```python
from build123d import *

# Parameters (mm, degrees)
SKETCH1_W           = 67
SKETCH1_H           = 40
BOSS_EXTRUDE1_DEPTH = 2
SKETCH2_W           = 55
SKETCH2_H           = 40
BOSS_EXTRUDE2_DEPTH = 2
SKETCH3_W           = 49
SKETCH3_H           = 38
BOSS_EXTRUDE4_DEPTH = 1
CUT_EXTRUDE1_REACH  = 80.09
SKETCH4_R           = 1.5
CUT_EXTRUDE2_REACH  = 80.09
SKETCH5_R           = 1.5
CUT_EXTRUDE3_REACH  = 80.09
SKETCH6_R           = 1.5
CUT_EXTRUDE4_REACH  = 80.09
SKETCH7_R           = 1.5
SKETCH9_W           = 2.5
SKETCH9_H           = 25
BOSS_EXTRUDE7_DEPTH = 15


with BuildPart() as part:
    # Sketch1 → Boss-Extrude1 (new body)
    with BuildSketch(Plane(origin=(0, 0, 0), x_dir=(1, 0, 0), z_dir=(0, 1, 0))):
        with Locations((33.5, 20)):
            Rectangle(SKETCH1_W, SKETCH1_H)
    extrude(amount=BOSS_EXTRUDE1_DEPTH)

    # Sketch2 → Boss-Extrude2 (add)
    with BuildSketch(Plane(origin=(0, 2, 0), x_dir=(1, 0, 0), z_dir=(0, 1, 0))):
        with Locations((33.5, 20)):
            Rectangle(SKETCH2_W, SKETCH2_H)
    extrude(amount=BOSS_EXTRUDE2_DEPTH)

    # Sketch3 → Boss-Extrude4 (add)
    with BuildSketch(Plane(origin=(0, 4, 0), x_dir=(1, 0, 0), z_dir=(0, 1, 0))):
        with Locations((35.5, 20)):
            Rectangle(SKETCH3_W, SKETCH3_H)
    extrude(amount=BOSS_EXTRUDE4_DEPTH)

    # Sketch4 → Cut-Extrude1 (cut, up to next)
    with BuildSketch(Plane(origin=(0, 2, 0), x_dir=(1, 0, 0), z_dir=(0, 1, 0)), mode=Mode.PRIVATE) as cut_extrude1_sk1:
        with Locations(Location((2.5, 37.5, 0), (0, 0, 270))):
            Circle(SKETCH4_R)
    cut_extrude1_tool1 = extrude(cut_extrude1_sk1.sketch, amount=-CUT_EXTRUDE1_REACH, mode=Mode.PRIVATE) & part.part
    add(cut_extrude1_tool1.solids().sort_by_distance((2.5, 2, -37.5))[0], mode=Mode.SUBTRACT)

    # Sketch5 → Cut-Extrude2 (cut, up to next)
    with BuildSketch(Plane(origin=(0, 2, 0), x_dir=(1, 0, 0), z_dir=(0, 1, 0)), mode=Mode.PRIVATE) as cut_extrude2_sk1:
        with Locations(Location((2.5, 2.5, 0), (0, 0, 270))):
            Circle(SKETCH5_R)
    cut_extrude2_tool1 = extrude(cut_extrude2_sk1.sketch, amount=-CUT_EXTRUDE2_REACH, mode=Mode.PRIVATE) & part.part
    add(cut_extrude2_tool1.solids().sort_by_distance((2.5, 2, -2.5))[0], mode=Mode.SUBTRACT)

    # Sketch6 → Cut-Extrude3 (cut, up to next)
    with BuildSketch(Plane(origin=(0, 2, 0), x_dir=(1, 0, 0), z_dir=(0, 1, 0)), mode=Mode.PRIVATE) as cut_extrude3_sk1:
        with Locations(Location((64.5, 37.5, 0), (0, 0, 270))):
            Circle(SKETCH6_R)
    cut_extrude3_tool1 = extrude(cut_extrude3_sk1.sketch, amount=-CUT_EXTRUDE3_REACH, mode=Mode.PRIVATE) & part.part
    add(cut_extrude3_tool1.solids().sort_by_distance((64.5, 2, -37.5))[0], mode=Mode.SUBTRACT)

    # Sketch7 → Cut-Extrude4 (cut, up to next)
    with BuildSketch(Plane(origin=(0, 2, 0), x_dir=(1, 0, 0), z_dir=(0, 1, 0)), mode=Mode.PRIVATE) as cut_extrude4_sk1:
        with Locations(Location((64.5, 2.5, 0), (0, 0, 270))):
            Circle(SKETCH7_R)
    cut_extrude4_tool1 = extrude(cut_extrude4_sk1.sketch, amount=-CUT_EXTRUDE4_REACH, mode=Mode.PRIVATE) & part.part
    add(cut_extrude4_tool1.solids().sort_by_distance((64.5, 2, -2.5))[0], mode=Mode.SUBTRACT)

    # Sketch9 → Boss-Extrude7 (add)
    with BuildSketch(Plane(origin=(0, 0, 0), x_dir=(-1, 0, 0), z_dir=(0, -1, 0))):
        with Locations((-1.25, 21.5)):
            Rectangle(SKETCH9_W, SKETCH9_H)
    extrude(amount=BOSS_EXTRUDE7_DEPTH)


solid = part.part
```
The listing builds one solid part. Answer for the finished solid, in the listing's coordinates (mm). A direction names the side the tool comes from. Round coordinates to 2 decimals unless told otherwise and drop trailing zeros. Order: outer loops, then holes, each group sorted by start corner. A loop starts at its lowest first (then second) coordinate and runs counter-clockwise, first axis right, second up. Notation, with made-up numbers: (-18, 62) -> (21, 62) arc R28 cw to (21, 90) -> close; hole circle Ø4 at (40, 45). An arc over 180 degrees is marked (long way). Answer as CSV lines item,"result". Start each with the question number.
(1) Flat-ended cylindrical pins translate along their axes: pin 1 Ø0.8 at (y, z) = (4.5, -25) entering from +X; pin 2 Ø0.8 at (x, y) = (41, 4.5) entering from -Z; pin 3 Ø2 at (x, y) = (1, -4.5) entering from -Z; pin 4 Ø2.5 at (x, z) = (64.5, -37.5) entering from -Y. Find the tip coordinate at first contact, or state that the pin passes through.
(2) For a pull along Z with two mould halves and no side action, classify faces 6 (the face through (1, -7, -9)), 7 (the face through (2.5, -7, -21)), 8 (the face through (65.987, 1.014, -37.695)) as +Z half, -Z half, draft (parallel to the pull), parting line (faces both ways), or undercut.
(3) A tool of negligible diameter and unlimited length cuts with its end or side. For faces 1 (the face through (61, 3, -20)), 2 (the face through (6, 3, -20)), 3 (the face through (33, 2, -40)), 4 (the face through (1, -7, -34)), 5 (the face through (35, 5, -20)), from which of +Z, -Z, +X, -X, +Y, -Y can it reach the whole face along a straight path? Write none if from no direction.
(4) The part is cut by section C-C (x = 48.5). Determine the outline of the cut face in (y, z).
(5) The part is cut by section A-A (z = -37.5). Determine the outline of the cut face in (x, y), then the cut area to 3 significant figures.
(6) The part is cut by section D-D (z = -27.5). Determine the outline of the cut face in (x, y).
(7) The part is cut by section B-B (x = 64.5). Determine the outline of the cut face in (y, z).
(8) Find the intervals of material crossed by probe 1 along X at (y, z) = (1.5, -2.5); probe 2 along Z at (x, y) = (64.5, 1.15); probe 3 along Y at (x, z) = (3, -31), in increasing order. Write a range as from..to.
Evaluation:
1,pin 1,"x = 60"
1,pin 2,"z = -39"
1,pin 3,"z = -34"
1,pin 4,"through"
2,face 6,"+Z half"
2,face 7,"draft"
2,face 8,"undercut"
3,face 1,"+Z, -Z, +X, +Y"
3,face 2,"+Z, -Z, -X, +Y"
3,face 3,"-Z, +X, -X, +Y, -Y"
3,face 4,"-Z, +X, -X, -Y"
3,face 5,"+Z, -Z, +X, -X, +Y"
4,outline,"(0, -40) -> (4, -40) -> (4, -39) -> (5, -39) -> (5, -1) -> (4, -1) -> (4, 0) -> (0, 0) -> close"
5,outline,"(0, 0) -> (1, 0) -> (1, 2) -> (0, 2) -> close; (4, 0) -> (63, 0) -> (63, 2) -> (61, 2) -> (61, 4) -> (60, 4) -> (60, 5) -> (11, 5) -> (11, 4) -> (6, 4) -> (6, 2) -> (4, 2) -> close; (66, 0) -> (67, 0) -> (67, 2) -> (66, 2) -> close"
5,area,"281 mm²"
6,outline,"(0, -15) -> (2.5, -15) -> (2.5, 0) -> (67, 0) -> (67, 2) -> (61, 2) -> (61, 4) -> (60, 4) -> (60, 5) -> (11, 5) -> (11, 4) -> (6, 4) -> (6, 2) -> (0, 2) -> close"
7,outline,"(0, -40) -> (2, -40) -> (2, -39) -> (0, -39) -> close; (0, -36) -> (2, -36) -> (2, -4) -> (0, -4) -> close; (0, -1) -> (2, -1) -> (2, 0) -> (0, 0) -> close"
8,probe 1,"0..1, 4..63, 66..67"
8,probe 2,"-40..-39, -36..-4, -1..0"
8,probe 3,"0..2"
